from build123d import *

# Parameters (mm, degrees)
EXTRUDE1_DEPTH     = 12.7
SKETCH2_W          = 50.8
SKETCH2_H          = 43.18
CUT_EXTRUDE1_DEPTH = 172.656838198
FILLET1_R          = 6.35


with BuildPart() as part:
    # Sketch1 → Extrude1 (new body)
    with BuildSketch(Plane.XY):
        Polygon((-95.25, 142.24), (95.25, 142.24), (95.25, 12.7), (53.975, 12.7), (53.975, 0), (34.925, 0), (34.925, 12.7), (-34.925, 12.7), (-34.925, 0), (-53.975, 0), (-53.975, 12.7), (-95.25, 12.7), align=None)
    extrude(amount=-EXTRUDE1_DEPTH)

    # Sketch2 → Cut-Extrude1 (cut, through all)
    with BuildSketch(Plane.XY):
        with Locations((0, 120.65)):
            Rectangle(SKETCH2_W, SKETCH2_H)
    extrude(amount=-CUT_EXTRUDE1_DEPTH, mode=Mode.SUBTRACT)

    # Fillet1
    fillet1_edges = [part.edges().sort_by_distance(p)[0] for p in [
        (-25.4, 99.06, -6.35),
        (25.4, 99.06, -6.35),
    ]]
    fillet(fillet1_edges, radius=FILLET1_R)


solid = part.part
The listing builds one solid part. Answer for the finished solid, in the listing's coordinates (mm). A direction names the side the tool comes from. Give positions to 0.01 mm unless a question says otherwise; leave off trailing zeros. Write each loop counter-clockwise with the first axis right and the second up, starting at its lowest first coordinate (ties: lowest second). Pieces come first, ordered by that corner, then holes.
Item 1: Determine the mould class of faces 1 (the flat face through (1, 72, 0)), 2 (the cylindrical face through (23.59, 100.97, -6.44)), 3 (the flat face through (34.925, 6, -6)), 4 (the flat face through (-53.975, 6, -6)) for opening direction X: released by +X, released by -X, zero draft, split by the parting line, or undercut.
Item 2: Section B-B, the plane x = -59.5 is taken. Write down the section's boundary in (y, z), plus the area to 3 significant figures.
Item 3: Flat-ended cylindrical pins translate along their axes: P1, Ø6.5, axis at y = 3, z = -4, coming from the +X side (3 decimals); P2, Ø6.5, axis at x = -4.5, z = -6.5, coming from the +Y side; P3, Ø4, axis at x = -17, z = -6, coming from the -Y side. Find the tip coordinate at first contact, or state that the pin passes through.
Item 4: Which of the six approach directions +Z, -Z, +X, -X, +Y, -Y give full straight-line access (tool end or side, diameter ignored) to faces 5 (the cylindrical face through (-23.59, 100.97, -6.44)), 6 (the flat face through (-61, 142.24, -6)), 7 (the flat face through (95.25, 78, -6)), 8 (the flat face through (53.975, 6, -6)), 9 (the flat face through (-74, 12.7, -6))?
Item 5: Find the intervals of material crossed by line 1 along X through (y, z) = (12, -2.25) (3 decimals); line 2 along Y through (x, z) = (-60, -12); line 3 along Y through (x, z) = (-9, -3.5), in increasing order.
Item 6: Section A-A, the plane z = -2 is taken. Write down the section's boundary in (x, y) (3 decimals).
Completed:
1. face 1: zero draft
1. face 2: undercut
1. face 3: undercut
1. face 4: released by -X
2. outline: (12.7, -12.7) - (142.24, -12.7) - (142.24, 0) - (12.7, 0) - close
2. area: 1,650 mm2
3. P1: stops at x = 53.975
3. P2: stops at y = 99.06
3. P3: stops at y = 12.7
4. face 5: +Z, -Z, +Y
4. face 6: +Z, -Z, +X, -X, +Y
4. face 7: +Z, -Z, +X, +Y, -Y
4. face 8: +Z, -Z, +X, -Y
4. face 9: +Z, -Z, -X, -Y
5. line 1: x = -53.975 to -34.925, 34.925 to 53.975
5. line 2: y = 12.7 to 142.24
5. line 3: y = 12.7 to 99.06
6. outline: (-95.25, 12.7) - (-53.975, 12.7) - (-53.975, 0) - (-34.925, 0) - (-34.925, 12.7) - (34.925, 12.7) - (34.925, 0) - (53.975, 0) - (53.975, 12.7) - (95.25, 12.7) - (95.25, 142.24) - (25.4, 142.24) - (25.4, 105.41) arc R6.35 cw to (19.05, 99.06) - (-19.05, 99.06) arc R6.35 cw to (-25.4, 105.41) - (-25.4, 142.24) - (-95.25, 142.24) - close
